from build123d import *

# Parameters (mm, degrees)
SKETCH1_W           = 7
SKETCH1_H           = 30
BOSS_EXTRUDE1_DEPTH = 3
SKETCH2_R           = 1.5
CUT_EXTRUDE1_DEPTH  = 3
SKETCH3_W           = 7
SKETCH3_H           = 8.5
BOSS_EXTRUDE2_DEPTH = 23
SKETCH4_R           = 1.5
CUT_EXTRUDE3_DEPTH  = 12
SKETCH5_W           = 7
SKETCH5_H           = 1
BOSS_EXTRUDE3_DEPTH = 1


with BuildPart() as part:
    # Sketch1 → Boss-Extrude1 (new body)
    with BuildSketch(Plane(origin=(0, 0, 0), x_dir=(1, 0, 0), z_dir=(0, 1, 0))):
        with Locations((-3.5, 15)):
            Rectangle(SKETCH1_W, SKETCH1_H)
    extrude(amount=BOSS_EXTRUDE1_DEPTH)

    # Sketch2 → Cut-Extrude1 (cut)
    with BuildSketch(Plane(origin=(0, 3, 0), x_dir=(1, 0, 0), z_dir=(0, 1, 0))):
        with Locations(Location((-3.5, 26.5, 0), (0, 0, 270))):
            Circle(SKETCH2_R)
        with Locations(Location((-3.5, 3.5, 0), (0, 0, 270))):
            Circle(SKETCH2_R)
    extrude(amount=-CUT_EXTRUDE1_DEPTH, mode=Mode.SUBTRACT)

    # Sketch3 → Boss-Extrude2 (add)
    with BuildSketch(Plane(origin=(0, 3, 0), x_dir=(1, 0, 0), z_dir=(0, 1, 0))):
        with Locations((-3.5, 19.25)):
            Rectangle(SKETCH3_W, SKETCH3_H)
        with Locations((-3.5, 10.75)):
            Rectangle(SKETCH3_W, SKETCH3_H)
    extrude(amount=BOSS_EXTRUDE2_DEPTH)

    # Sketch4 → Cut-Extrude3 (cut)
    with BuildSketch(Plane(origin=(0, 26, 0), x_dir=(1, 0, 0), z_dir=(0, 1, 0))):
        with Locations(Location((-3.5, 15, 0), (0, 0, 270))):
            Circle(SKETCH4_R)
    extrude(amount=-CUT_EXTRUDE3_DEPTH, mode=Mode.SUBTRACT)

    # Sketch5 → Boss-Extrude3 (add)
    with BuildSketch(Plane(origin=(0, 26, 0), x_dir=(1, 0, 0), z_dir=(0, 1, 0))):
        with Locations((-3.5, 23)):
            Rectangle(SKETCH5_W, SKETCH5_H)
        with Locations((-3.5, 7)):
            Rectangle(SKETCH5_W, SKETCH5_H)
    extrude(amount=BOSS_EXTRUDE3_DEPTH)


solid = part.part
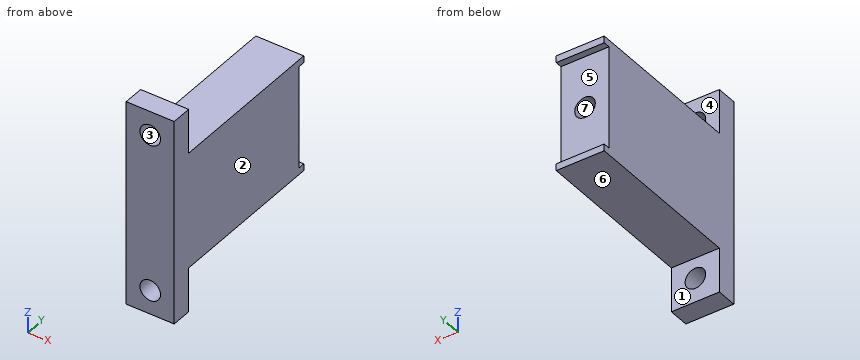
Geometry: final body of the model. Coordinates: model frame, mm. Face numbers are marked on the shaded views. A direction names the side the tool comes from. Coordinates: 2 decimals unless noted, no trailing zeros. Loops run counter-clockwise (first coordinate to the right, second up) from the corner with the lowest first, then second, coordinate; pieces in that order, holes last. Notation, with made-up numbers: (9.25, -7.5) - (15.25, -7.5) arc R13 ccw to (15.25, 6.5) - close; hole circle Ø5 at (49.5, -21). An arc over 180 degrees is marked (long way). Put each result on its own line as item: value. Start each with the question number.
Q1. Set-up query: the marked faces 4, 5, 6 and 7. Return all of +Z, -Z, +X, -X, +Y, -Y with unobstructed straight access to the full face (end or side cutting, diameter ignored); none if empty.
Q2. Line query: line 1 (X direction, y = 18.5, z = -15); line 2 (Y direction, x = -4, z = -28.5); line 3 (Y direction, x = -4.5, z = -19.25). Output: solid intervals per line, ascending.
Q3. Cut plane C-C, the plane y = 24.25. Return loops of the section in (x, z), and give its area (3 significant figures).
Q4. Cut plane D-D, the plane x = -0.5. Return loops of the section in (y, z), and give its area (3 significant figures).
Q5. Cut plane B-B, the plane z = -26.5. Return loops of the section in (x, y), and give its area (3 significant figures).
Q6. Pin query (flat end, axial travel): pin 1 Ø1.5 at (x, y) = (-3.5, 11.5) entering from +Z; pin 2 Ø3.5 at (x, y) = (-3, 20.5) entering from -Z; pin 3 Ø3.5 at (x, z) = (-3, -18) entering from +Y. Return the tip coordinate at first contact, or that it passes through.
Q7. Pull-direction query (X, two-part tool) for the marked faces 1, 2 and 3; classes: released by +X, released by -X, zero draft, split by the parting line, or undercut.
Q8. Cut plane A-A, the plane x = -3.5. Return loops of the section in (y, z).
Filled sheet:
1. face 4: +Z, +X, -X, +Y
1. face 5: +X, -X, +Y
1. face 6: -Z, +X, -X, +Y
1. face 7: +Y
2. line 1: -7 to -5, -2 to 0
2. line 2: 0 to 3
2. line 3: 0 to 26
3. outline: (-7, -23.5) - (0, -23.5) - (0, -6.5) - (-7, -6.5) - close; hole circle Ø3 at (-3.5, -15)
3. area: 112 mm²
4. outline: (0, -30) - (3, -30) - (3, -23.5) - (27, -23.5) - (27, -22.5) - (26, -22.5) - (26, -7.5) - (27, -7.5) - (27, -6.5) - (3, -6.5) - (3, 0) - (0, 0) - close
4. area: 483 mm²
5. outline: (-7, 0) - (-5, 0) - (-5, 3) - (-7, 3) - close; (-2, 0) - (0, 0) - (0, 3) - (-2, 3) - close
5. area: 12.0 mm²
6. pin 1: z = -6.5
6. pin 2: z = -23.5
6. pin 3: y = 26
7. face 1: zero draft
7. face 2: released by +X
7. face 3: undercut
8. outline: (0, -30) - (3, -30) - (3, -28) - (0, -28) - close; (0, -25) - (3, -25) - (3, -23.5) - (27, -23.5) - (27, -22.5) - (26, -22.5) - (26, -16.5) - (14, -16.5) - (14, -13.5) - (26, -13.5) - (26, -7.5) - (27, -7.5) - (27, -6.5) - (3, -6.5) - (3, -5) - (0, -5) - close; (0, -2) - (3, -2) - (3, 0) - (0, 0) - close
